from build123d import *

# Parameters (mm, degrees)
BOSS_EXTRUDE1_DEPTH = 25
SKETCH2_W           = 3.2
SKETCH2_H           = 9.5
CUT_EXTRUDE1_DEPTH  = 55.5
SKETCH3_R           = 2.75
CUT_EXTRUDE2_DEPTH  = 37
CUT_EXTRUDE3_DEPTH  = 17
SKETCH9_W           = 6.2
SKETCH9_H           = 19.95
CUT_EXTRUDE8_DEPTH  = 18
SKETCH10_R          = 2.75
BOSS_EXTRUDE2_DEPTH = 0.2
SKETCH11_R          = 2.75
BOSS_EXTRUDE3_DEPTH = 0.2
SKETCH12_R          = 1.6
BOSS_EXTRUDE4_DEPTH = 4


with BuildPart() as part:
    # Sketch1 → Boss-Extrude1 (new body)
    with BuildSketch(Plane.XY):
        with BuildLine():
            Line((0, 2.395761144), (-1.762956434, 2.395761144))
            ThreePointArc((-1.762956434, 2.395761144), (-2.146371288, 2.574835842), (-2.255146546, 2.983788945))
            Line((-2.255146546, 2.983788945), (-1.936807424, 4.763719442))
            ThreePointArc((-1.936807424, 4.763719442), (-2.424010325, 5.602484354), (-3.331198308, 5.259113989))
            Line((-3.331198308, 5.259113989), (-5, 2.245761144))
            Line((-5, 2.245761144), (-5, 0.895761144))
            Line((-5, 0.895761144), (0, 0.895761144))
            Line((0, 0.895761144), (0, -0.895761144))
            Line((0, -0.895761144), (-5, -0.895761144))
            Line((-5, -0.895761144), (-5, -2.245761144))
            Line((-5, -2.245761144), (-3.331198308, -5.259113989))
            ThreePointArc((-3.331198308, -5.259113989), (-2.424010325, -5.602484354), (-1.936807424, -4.763719442))
            Line((-1.936807424, -4.763719442), (-2.255146546, -2.983788945))
            ThreePointArc((-2.255146546, -2.983788945), (-2.146371288, -2.574835842), (-1.762956434, -2.395761144))
            Line((-1.762956434, -2.395761144), (0, -2.395761144))
            Line((0, -2.395761144), (0, -9.975))
            Line((0, -9.975), (18, -9.975))
            Line((18, -9.975), (18, 9.975))
            Line((18, 9.975), (0, 9.975))
            Line((0, 9.975), (0, 2.395761144))
        make_face()
    extrude(amount=BOSS_EXTRUDE1_DEPTH)

    # Sketch2 → Cut-Extrude1 (cut, symmetric)
    with BuildSketch(Plane.ZY):
        with Locations((20.4, 0)):
            Rectangle(SKETCH2_W, SKETCH2_H)
    extrude(amount=CUT_EXTRUDE1_DEPTH, both=True, mode=Mode.SUBTRACT)

    # Sketch3 → Cut-Extrude2 (cut)
    with BuildSketch(Plane.XY.offset(25)):
        with Locations((5.1, -0.01)):
            Circle(SKETCH3_R)
    extrude(amount=-CUT_EXTRUDE2_DEPTH, mode=Mode.SUBTRACT)

    # Sketch4 → Cut-Extrude3 (cut)
    with BuildSketch(Plane(origin=(0, 0, 0), x_dir=(-1, 0, 0), z_dir=(0, 0, -1))):
        Polygon((-10.555960044, -0.01), (-7.827980022, -4.735), (-2.372019978, -4.735), (0.355960044, -0.01), (-2.372019978, 4.715), (-7.827980022, 4.715), align=None)
    extrude(amount=-CUT_EXTRUDE3_DEPTH, mode=Mode.SUBTRACT)

    # Sketch9 → Cut-Extrude8 (cut)
    with BuildSketch(Plane.ZY):
        with Locations((21.9, 0)):
            Rectangle(SKETCH9_W, SKETCH9_H)
    extrude(amount=CUT_EXTRUDE8_DEPTH, mode=Mode.SUBTRACT)

    # Sketch10 → Boss-Extrude2 (add)
    with BuildSketch(Plane(origin=(0, 0, 17), x_dir=(-1, 0, 0), z_dir=(0, 0, -1))):
        with Locations((-5.1, -0.01)):
            Circle(SKETCH10_R)
    extrude(amount=-BOSS_EXTRUDE2_DEPTH)

    # Sketch11 → Boss-Extrude3 (add)
    with BuildSketch(Plane(origin=(0, 0, 22), x_dir=(-1, 0, 0), z_dir=(0, 0, -1))):
        with Locations((-5.1, -0.01)):
            Circle(SKETCH11_R)
    extrude(amount=-BOSS_EXTRUDE3_DEPTH)

    # Sketch12 → Boss-Extrude4 (add)
    with BuildSketch(Plane(origin=(0, 0, 0), x_dir=(-1, 0, 0), z_dir=(0, 0, -1))):
        with BuildLine():
            Line((-10, 4.48373582), (-12, 0))
            Line((-12, 0), (-10, -4.48373582))
            Line((-10, -4.48373582), (-10, -13.975))
            ThreePointArc((-10, -13.975), (-14.5, -18.475), (-19, -13.975))
            Line((-19, -13.975), (-19, 13.975))
            ThreePointArc((-19, 13.975), (-14.5, 18.475), (-10, 13.975))
            Line((-10, 13.975), (-10, 4.48373582))
        make_face()
        with Locations((-14.5, -13.975)):
            Circle(SKETCH12_R, mode=Mode.SUBTRACT)
        with Locations((-14.5, 13.975)):
            Circle(SKETCH12_R, mode=Mode.SUBTRACT)
    extrude(amount=-BOSS_EXTRUDE4_DEPTH)


solid = part.part
Source: CAD feature listing. Evaluate the final solid. Frame: model axes, mm. A direction names the side the tool comes from. Round coordinates to 2 decimals unless told otherwise and drop trailing zeros. Write each loop counter-clockwise with the first axis right and the second up, starting at its lowest first coordinate (ties: lowest second). Pieces come first, ordered by that corner, then holes. Notation, with made-up numbers: M -30.5,89.5 L 1.5,89.5 A33 ccw 1.5,126.5 Z; hole C 70,88 d11. An arc over 180 degrees is marked long. One line per item, written item: value. Start each with the question number.
Item 1: Section query A-A (x = 14.5). Return the cut outline in (y, z) (3 decimals).
Item 2: Section query B-B (x = 5.1). Return the cut outline in (y, z) (3 decimals).
Item 3: Set-up query: faces 4 (the flat face through (-3, 0.896, 9)), 5 (the flat face through (5, 0, 22.2)), 6 (the flat face through (1.17, 2.63, 8.38)), 7 (the flat face through (-1, -2.396, 9)), 8 (the flat face through (-2.094, -3.886, 9.268)). Return all of +Z, -Z, +X, -X, +Y, -Y with unobstructed straight access to the full face (end or side cutting, diameter ignored); none if empty.
Item 4: Section query D-D (z = 9.5). Return the cut outline in (x, y) (3 decimals), plus the area to 3 significant figures.
Item 5: Pin query (flat end, axial travel): pin 1 (3 mm diameter, centred on x = 5.5, z = 11, fed in from -Y) (3 decimals); pin 2 (8 mm diameter, centred on x = 0, y = 9.5, fed in from -Z); pin 3 (4.5 mm diameter, centred on x = 4, y = -1.5, fed in from -Z); pin 4 (5.5 mm diameter, centred on x = -3.5, z = 10.5, fed in from -Y). Return the tip coordinate at first contact, or that it passes through.
Item 6: Mould query, pull axis Y, two halves, no side actions, for faces 1 (the flat face through (19, 0, 2)), 2 (the cylindrical face through (14.401, -18.474, 1.972)), 3 (the flat face through (5, 4.715, 8)). Classes: pulls with the +Y half, pulls with the -Y half, needs draft (parallel to the pull), parting line crosses it, or undercut.
Item 7: Ray query, L1, parallel to Y at x = 14.5, z = 1.4 (3 decimals); L2, parallel to Z at x = 8.25, y = 1.5; L3, parallel to Z at x = 16.25, y = -1. Return the intervals inside material, ascending. Write a range as from..to.
Item 8: Section query C-C (z = 3.5). State how many separate pieces and enclosed holes the cut face has, plus the area to 3 significant figures.
Result set:
1. outline: M -18.475,0 L -15.575,0 L -15.575,4 L -18.475,4 Z; M -12.375,0 L 12.375,0 L 12.375,4 L 9.975,4 L 9.975,25 L -9.975,25 L -9.975,4 L -12.375,4 Z; M 15.575,0 L 18.475,0 L 18.475,4 L 15.575,4 Z; hole M -4.75,18.8 L 4.75,18.8 L 4.75,22 L -4.75,22 Z
2. outline: M -9.975,0 L -4.735,0 L -4.735,17 L 4.715,17 L 4.715,0 L 9.975,0 L 9.975,25 L 2.74,25 L 2.74,22.2 L -2.76,22.2 L -2.76,25 L -9.975,25 Z; hole M -4.75,18.8 L -2.76,18.8 L -2.76,17.2 L 2.74,17.2 L 2.74,18.8 L 4.75,18.8 L 4.75,22 L -4.75,22 Z
3. face 4: +Z, -Z, -X
3. face 5: +Z
3. face 6: -Z
3. face 7: +Z, -Z, -Y
3. face 8: +Z, -Z
4. outline: M -5,-2.246 L -3.331,-5.259 A0.75 ccw -1.937,-4.764 L -2.255,-2.984 A0.5 cw -1.763,-2.396 L 0,-2.396 L 0,-9.975 L 18,-9.975 L 18,9.975 L 0,9.975 L 0,2.396 L -1.763,2.396 A0.5 cw -2.255,2.984 L -1.937,4.764 A0.75 ccw -3.331,5.259 L -5,2.246 L -5,0.896 L 0,0.896 L 0,0.607 L 2.372,4.715 L 7.828,4.715 L 10.556,-0.01 L 7.828,-4.735 L 2.372,-4.735 L 0,-0.627 L 0,-0.896 L -5,-0.896 Z
4. area: 309 mm²
5. pin 1: stops at y = -9.975
5. pin 2: stops at z = 0
5. pin 3: stops at z = 17
5. pin 4: stops at y = -5.65
6. face 1: needs draft
6. face 2: pulls with the -Y half
6. face 3: undercut
7. L1: y = -18.475..-15.575, -12.375..12.375, 15.575..18.475
7. L2: z = 17..18.8, 22..25
7. L3: z = 0..18.8, 22..25
8. separate pieces: 1
8. enclosed holes: 2
8. area: 449 mm²
